Read the model definition and answer for the solid it produces. Units are mm, in the model's axes. A direction names the side the tool comes from. Round coordinates to 2 decimals unless told otherwise and drop trailing zeros. Order: outer loops, then holes, each group sorted by start corner. A loop starts at its lowest first (then second) coordinate and runs counter-clockwise, first axis right, second up. Notation, with made-up numbers: (-10, 52.25) -> (39, 52.25) arc R22 ccw to (39, 91.25) -> close; hole circle Ø10 at (35, 82.25). An arc over 180 degrees is marked (long way). Use a Markdown table: item, result. Add a question column.
1. The mould has two halves that part along X. Classify faces 1 (the face through (114.72, 25.04, 9.13)), 2 (the face through (7.51, -216.53, 8.87)), 3 (the face through (64, 0, 12)): +X half, -X half, draft (parallel to the pull), parting line (faces both ways), or undercut.
2. Given pin 1 (1.5 mm diameter, centred on y = -130, z = 5.5, fed in from +X); pin 2 (14.5 mm diameter, centred on x = 55, y = -2.5, fed in from +Z); pin 3 (3.5 mm diameter, centred on x = 55.5, z = 11.5, fed in from +Y); pin 4 (1.5 mm diameter, centred on x = 87.5, y = 143.5, fed in from -Z), each flat-ended and moving along its own axis, determine where each tip first touches the part or whether it passes through.
3. Section C-C, the plane x = 87 is taken. Give the vertices of the cut face in (y, z).
4. Consider L1, parallel to X at y = -15, z = 10; L2, parallel to Z at x = 47, y = -12.5; L3, parallel to X at y = -204.5, z = 14.5. Determine where each line is inside the solid, lowest interval first. Write a range as [from, to].
5. Section A-A, the plane z = 9 is taken. Give the vertices of the cut face in (x, y), then the cut area to 3 significant figures.
6. For faces 4 (the face through (55, 30, 12)), 5 (the face through (44, 3, 18)), determine the directions among +Z, -Z, +X, -X, +Y, -Y from which every point of the face is accessible in a straight line to the end or side of a thin tool.
7. Section B-B, the plane y = -75 is taken. Give the vertices of the cut face in (x, z), then the cut area to 3 significant figures.
```python
from build123d import *

# Parameters (mm, degrees)
PAD_DEPTH    = 18
SKETCH001_W  = 18
SKETCH001_H  = 60
POCKET_DEPTH = 12
CHAMFER_SIZE = 15
FILLET_R     = 5
FILLET001_R  = 15
FILLET002_R  = 50


with BuildPart() as part:
    # Sketch → Pad (new body)
    with BuildSketch(Plane.XY):
        Polygon((0, 225), (0, -225), (74.720813, -214.498675), (115, -25), (115, 25), (74.720813, 214.498675), align=None)
    extrude(amount=PAD_DEPTH)

    # Sketch001 → Pocket (cut)
    with BuildSketch(Plane.XY.offset(18)):
        with Locations((55, 0)):
            Rectangle(SKETCH001_W, SKETCH001_H)
    extrude(amount=-POCKET_DEPTH, mode=Mode.SUBTRACT)

    # Chamfer
    chamfer_edges = [part.edges().sort_by_distance(p)[0] for p in [
        (0, -225, 9),
        (0, 225, 9),
    ]]
    chamfer(chamfer_edges, length=CHAMFER_SIZE)

    # Fillet
    fillet_edges = [part.edges().sort_by_distance(p)[0] for p in [
        (14.854021, 222.912403, 9),
        (0, 210, 9),
        (0, -210, 9),
        (14.854021, -222.912403, 9),
    ]]
    fillet(fillet_edges, radius=FILLET_R)

    # Fillet001
    fillet001_edges = [part.edges().sort_by_distance(p)[0] for p in [
        (74.720813, -214.498675, 9),
        (74.720813, 214.498675, 9),
    ]]
    fillet(fillet001_edges, radius=FILLET001_R)

    # Fillet002
    fillet002_edges = [part.edges().sort_by_distance(p)[0] for p in [
        (115, -25, 9),
        (115, 25, 9),
    ]]
    fillet(fillet002_edges, radius=FILLET002_R)


solid = part.part
```
Verdict:
| question | item | result |
|---|---|---|
| 1 | face 1 | +X half |
| 1 | face 2 | -X half |
| 1 | face 3 | undercut |
| 2 | pin 1 | stops at x = 92.84 |
| 2 | pin 2 | stops at z = 6 |
| 2 | pin 3 | stops at y = 217.45 |
| 2 | pin 4 | stops at z = 0 |
| 3 | outline | (-156.73, 0) -> (156.73, 0) -> (156.73, 18) -> (-156.73, 18) -> close |
| 4 | L1 | x = [0, 46], [64, 115] |
| 4 | L2 | z = [0, 6] |
| 4 | L3 | x = [0, 76.84] |
| 5 | outline | (0, -207.72) arc R5 ccw to (1.72, -211.49) -> (13.13, -221.42) arc R5 ccw to (17.11, -222.6) -> (64.32, -215.96) arc R15 ccw to (76.9, -204.23) -> (113.91, -30.14) arc R50 ccw to (115, -19.74) -> (115, 19.74) arc R50 ccw to (113.91, 30.14) -> (76.9, 204.23) arc R15 ccw to (64.32, 215.96) -> (17.11, 222.6) arc R5 ccw to (13.13, 221.42) -> (1.72, 211.49) arc R5 ccw to (0, 207.72) -> close; hole (46, -30) -> (64, -30) -> (64, 30) -> (46, 30) -> close |
| 5 | area | 41,100 mm2 |
| 6 | face 4 | +Z |
| 6 | face 5 | +Z, +X, -X, +Y, -Y |
| 7 | outline | (0, 0) -> (104.37, 0) -> (104.37, 18) -> (0, 18) -> close |
| 7 | area | 1,880 mm2 |
